```python
from build123d import *

# Parameters (mm, degrees)
F0_R     = 12.7
F1_DEPTH = 19.05
F2_SIZE  = 3.175
F3_T     = -3.175
F4_SIZE  = 3.17499


# Not quite as in the source:
# - a fillet or chamfer is up to 0.001 mm smaller than in the source, because OpenCascade refuses the exact size


with BuildPart() as f1:
    # F0 (on Top) → F1 (new body)
    with BuildSketch(Plane.XY):
        Circle(F0_R)
    extrude(amount=F1_DEPTH)

    # F2
    f2_edges = [f1.edges().sort_by_distance(p)[0] for p in [
        (-12.7, 0, 19.05),
    ]]
    chamfer(f2_edges, length=F2_SIZE)

    # F3
    f3_openings = [f1.faces().sort_by_distance(p)[0] for p in [
        (0, 0, 0),
    ]]
    offset(amount=F3_T, openings=f3_openings)

    # F4 (size 3.175 in the source; OpenCascade refuses exactly that, so slightly less here)
    f4_edges = [f1.edges().sort_by_distance(p)[0] for p in [
        (-9.525, 0, 0),
    ]]
    chamfer(f4_edges, length=F4_SIZE)


solid = f1.part
```
Input: part model. Units: mm. Frame: model coordinates. A direction names the side the tool comes from. Give positions to 0.01 mm unless a question says otherwise; leave off trailing zeros. Order: outer loops, then holes, each group sorted by start corner. A loop starts at its lowest first (then second) coordinate and runs counter-clockwise, first axis right, second up. Notation, with made-up numbers: M -32,69 L 5,69 A18 cw 5,91 Z; hole C 43.5,67 d1. An arc over 180 degrees is marked long. Return JSON: item names as keys, results as strings.
Item 1: Pull-direction query (X, two-part tool) for faces 1 (the flat face through (0, 0, 15.875)), 2 (the cylindrical face through (-2.75, -12.4, 7.83)), 3 (the flat face through (0, 0, 19.05)); classes: +X half, -X half, draft (parallel to the pull), parting line (faces both ways), or undercut.
Solutions:
{"face 1": "undercut", "face 2": "parting line", "face 3": "draft"}
Item 2: Cut plane C-C (z = 4.5). Return loops of the section in (x, y) (3 decimals), then the cut area to 3 significant figures.
Solutions:
{"outline": "C 0,0 d25.4; hole C 0,0 d19.05", "area": "222 mm^2"}
Item 3: Access query for faces 4 (the conical face through (-9.67, 0.426, 18.896)), 5 (the cylindrical face through (-7.559, -5.796, 8.788)). Directions: +Z, -Z, +X, -X, +Y, -Y. A direction counts if a zero-diameter tool reaches every point of the face in a straight line with its end or side. Return the directions, or none.
Solutions:
{"face 4": "+Z", "face 5": "-Z"}
Item 4: Cut plane D-D (z = 18). Return loops of the section in (x, y) (3 decimals), then the cut area to 3 significant figures.
Solutions:
{"outline": "C 0,0 d21.15", "area": "351 mm^2"}
Item 5: First-contact query: P1, Ø1, axis at y = 9, z = 13, coming from the +X side; P2, Ø5, axis at x = -4, z = 6, coming from the +Y side; P3, Ø1.5, axis at x = -7.5, z = 12.5, coming from the +Y side. Flat tips, straight axial feed; report the tip coordinate or a pass-through.
Solutions:
{"P1": "x = 9.44", "P2": "y = 12.61", "P3": "y = 10.76"}
Item 6: Ray query, probe 1 along Y at (x, z) = (0, 5.75) (3 decimals); probe 2 along Y at (x, z) = (-8.75, 9.75); probe 3 along X at (y, z) = (-3.5, 15.5). Return the intervals inside material, ascending.
Solutions:
{"probe 1": "-12.7 to -9.525, 9.525 to 12.7", "probe 2": "-9.2 to -3.76, 3.76 to 9.2", "probe 3": "-12.21 to -7.84, 7.84 to 12.21"}
